from build123d import *

# Parameters (mm, degrees)
F0_R     = 1.63195
F0_R_2   = 0.8509
F1_DEPTH = 2.3876


with BuildPart() as f1:
    # F0 (on Front) → F1 (new body)
    with BuildSketch(Plane.XZ):
        with BuildLine():
            ThreePointArc((75.886587, 0), (74.956651, 2.245064), (72.711587, 3.175))
            Line((72.711587, 3.175), (6.036587, 3.175))
            ThreePointArc((6.036587, 3.175), (3.791523, 2.245064), (2.861587, 0))
            ThreePointArc((2.861587, 0), (3.791523, -2.245064), (6.036587, -3.175))
            Line((6.036587, -3.175), (72.711587, -3.175))
            ThreePointArc((72.711587, -3.175), (74.956651, -2.245064), (75.886587, 0))
        make_face()
        with Locations((6.036587, 0)):
            Circle(F0_R, mode=Mode.SUBTRACT)
        with Locations((72.711587, 0)):
            Circle(F0_R_2, mode=Mode.SUBTRACT)
    extrude(amount=-F1_DEPTH)


solid = f1.part
Design review of the part built by this model. Coordinates are the model's own, in mm. Give positions to 0.01 mm unless a question says otherwise; leave off trailing zeros. Loops run counter-clockwise (first coordinate to the right, second up) from the corner with the lowest first, then second, coordinate; pieces in that order, holes last. Notation, with made-up numbers: M -38,-9 L 4,-9 A14 ccw 4,0 Z; hole C 30,-5 d8. An arc over 180 degrees is marked long. Write item = value, one per line.
Q1. To check wall thickness, follow line 1 (X direction, y = 0.95, z = 1.25); line 2 (X direction, y = 0.95, z = -1.75). State the ranges of each line that lie inside material, in increasing order. Write a range as [from, to].
Output values:
line_1 = [3.12, 4.99], [7.09, 75.63]
line_2 = [3.39, 75.36]
Q2. Draft analysis for pull direction Z (two halves, no side actions). For faces 1 (the cylindrical face through (73.52, 1.18, 0.26)), 2 (the cylindrical face through (7.54, 1.18, -0.63)), 3 (the flat face through (40, 1, 3.175)), 4 (the flat face through (39, 2.388, 0)), state which applies: +Z half, -Z half, draft (parallel to the pull), parting line (faces both ways), or undercut.
Output values:
face_1 = undercut
face_2 = undercut
face_3 = +Z half
face_4 = draft
Q3. We need section B-B (z = -2.5). Give the boundary of the cut face in (x, y), plus the area to 3 significant figures.
Output values:
outline = M 4.08,0 L 74.67,0 L 74.67,2.39 L 4.08,2.39 Z
area = 169 mm^2
Q4. We need section A-A (z = 2.25). Give the boundary of the cut face in (x, y), plus the area to 3 significant figures.
Output values:
outline = M 3.8,0 L 74.95,0 L 74.95,2.39 L 3.8,2.39 Z
area = 170 mm^2
